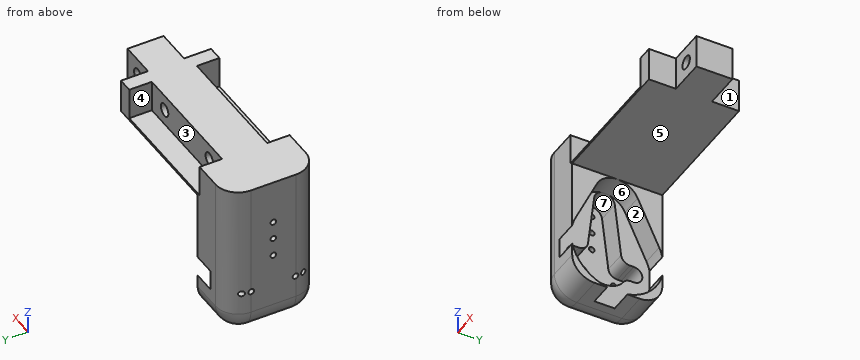
```python
from build123d import *

# Parameters (mm, degrees)
EXTRUDE_1_DEPTH      = 20
FILLET_1_R           = 5
SKETCH_2_R           = 8
CUT_EXTRUDE_1_DEPTH  = 5
SKETCH_3_R           = 6
CUT_EXTRUDE_2_DEPTH  = 1
CUT_EXTRUDE_3_DEPTH  = 5
CUT_EXTRUDE_4_DEPTH  = 5
SKETCH_6_R           = 0.625
CUT_EXTRUDE_5_DEPTH  = 4
SKETCH_7_W           = 27.5
SKETCH_7_H           = 5
CUT_EXTRUDE_6_DEPTH  = 7
SKETCH_8_R           = 1.45
CUT_EXTRUDE_7_DEPTH  = 12
CUT_EXTRUDE_8_DEPTH  = 6
CUT_EXTRUDE_START    = -20
CUT_EXTRUDE_9_DEPTH  = 6
SKETCH_13_W          = 12
SKETCH_13_H          = 27.5
CUT_EXTRUDE_10_DEPTH = 11
SKETCH_14_R          = 1.46
CUT_EXTRUDE_11_DEPTH = 11


with BuildPart() as part:
    # Эскиз1 → Бобышка-Вытянуть1 (new body)
    with BuildSketch(Plane(origin=(0, 0, 0), x_dir=(1, 0, 0), z_dir=(0, 1, 0))):
        Polygon((-13, 27.5), (-13, 0), (13, 0), (13, 27.5), (25, 27.5), (25, -7.5), (-25, -7.5), (-25, 27.5), align=None)
    extrude(amount=EXTRUDE_1_DEPTH)

    # Скругление1
    fillet_1_edges = [part.edges().sort_by_distance(p)[0] for p in [
        (19, 0, -27.5),
        (25, 10, -27.5),
        (-25, 10, -27.5),
        (-19, 20, -27.5),
        (-25, 20, -10),
        (25, 20, -10),
        (19, 20, -27.5),
        (25, 0, -10),
        (-25, 0, -10),
        (-19, 0, -27.5),
    ]]
    fillet(fillet_1_edges, radius=FILLET_1_R)

    # Эскиз2 → Вырез-Вытянуть1 (cut)
    with BuildSketch(Plane.ZY.offset(-13)):
        with Locations((-17.5, 10)):
            Circle(SKETCH_2_R)
    extrude(amount=-CUT_EXTRUDE_1_DEPTH, mode=Mode.SUBTRACT)

    # Эскиз3 → Вырез-Вытянуть2 (cut)
    with BuildSketch(Plane.ZY.offset(-18)):
        with Locations((-17.5, 10)):
            Circle(SKETCH_3_R)
    extrude(amount=-CUT_EXTRUDE_2_DEPTH, mode=Mode.SUBTRACT)

    # Эскиз4 → Вырез-Вытянуть3 (cut)
    with BuildSketch(Plane(origin=(-13, 0, 0), x_dir=(0, 0, -1), z_dir=(1, 0, 0))):
        with BuildLine():
            Line((13.195, 19.30212207), (2.9, 14.537620522))
            ThreePointArc((2.9, 14.537620522), (0, 10), (2.9, 5.462379478))
            Line((2.9, 5.462379478), (13.195, 0.69787793))
            ThreePointArc((13.195, 0.69787793), (27.75, 10), (13.195, 19.30212207))
        make_face()
    extrude(amount=-CUT_EXTRUDE_3_DEPTH, mode=Mode.SUBTRACT)

    # Эскиз5 → Вырез-Вытянуть4 (cut)
    with BuildSketch(Plane(origin=(-18, 0, 0), x_dir=(0, 0, -1), z_dir=(1, 0, 0))):
        with BuildLine():
            Line((19.4, 15.812916652), (19.4, 16.49838717))
            ThreePointArc((19.4, 16.49838717), (17.499999842, 18.39838717), (15.6, 16.498386854))
            Line((15.6, 16.498386854), (15.6, 15.665366642))
            ThreePointArc((15.6, 15.665366642), (15.094249889, 14.335999398), (13.832782732, 13.678959785))
            Line((13.832782732, 13.678959785), (1.932299859, 12.284367885))
            ThreePointArc((1.932299859, 12.284367885), (-0.1, 10), (1.932299859, 7.715632115))
            Line((1.932299859, 7.715632115), (13.832782732, 6.321040215))
            ThreePointArc((13.832782732, 6.321040215), (15.094249889, 5.664000602), (15.6, 4.334633358))
            Line((15.6, 4.334633358), (15.6, 3.501613146))
            ThreePointArc((15.6, 3.501613146), (17.5, 1.601613146), (19.4, 3.501613146))
            Line((19.4, 3.501613146), (19.4, 4.187083665))
            ThreePointArc((19.4, 4.187083665), (19.635266181, 5.128207436), (20.285714286, 5.847916677))
            ThreePointArc((20.285714286, 5.847916677), (22.5, 10), (20.285714286, 14.152083323))
            ThreePointArc((20.285714286, 14.152083323), (19.635266107, 14.871792704), (19.4, 15.812916652))
        make_face()
    extrude(amount=-CUT_EXTRUDE_4_DEPTH, mode=Mode.SUBTRACT)

    # Эскиз6 → Вырез-Вытянуть5 (cut)
    with BuildSketch(Plane(origin=(-23, 0, 0), x_dir=(0, 0, -1), z_dir=(1, 0, 0))):
        with Locations((2.278018202, 10)):
            Circle(SKETCH_6_R)
        with Locations((6.311115384, 10)):
            Circle(SKETCH_6_R)
        with Locations((10.428235425, 10)):
            Circle(SKETCH_6_R)
        with Locations((17.5, 14.907931149)):
            Circle(SKETCH_6_R)
        with Locations((17.5, 16.848859168)):
            Circle(SKETCH_6_R)
        with Locations((17.5, 5.082068851)):
            Circle(SKETCH_6_R)
        with Locations((17.5, 3.141140832)):
            Circle(SKETCH_6_R)
    extrude(amount=-CUT_EXTRUDE_5_DEPTH, mode=Mode.SUBTRACT)

    # Эскиз7 → Вырез-Вытянуть6 (cut)
    with BuildSketch(Plane.XY.offset(7.5)):
        with Locations((0, 17.5)):
            Rectangle(SKETCH_7_W, SKETCH_7_H)
        with Locations((0, 2.5)):
            Rectangle(SKETCH_7_W, SKETCH_7_H)
    extrude(amount=-CUT_EXTRUDE_6_DEPTH, mode=Mode.SUBTRACT)

    # Эскиз8 → Вырез-Вытянуть7 (cut)
    with BuildSketch(Plane(origin=(0, 15, 0), x_dir=(1, 0, 0), z_dir=(0, 1, 0))):
        with Locations(Location((-8.75, -4, 0), (0, 0, 270))):
            Circle(SKETCH_8_R)
        with Locations(Location((8.75, -4, 0), (0, 0, 270))):
            Circle(SKETCH_8_R)
    extrude(amount=-CUT_EXTRUDE_7_DEPTH, mode=Mode.SUBTRACT)

    # Эскиз11 → Вырез-Вытянуть8 (cut)
    with BuildSketch(Plane(origin=(0, 20, 0), x_dir=(1, 0, 0), z_dir=(0, 1, 0))):
        Polygon((13, 27.5), (13, 0), (17, 0), (17, -7.5), (25, -7.5), (25, 27.5), align=None)
    extrude(amount=-CUT_EXTRUDE_8_DEPTH, mode=Mode.SUBTRACT)

    # Эскиз11<2> → Вырез-Вытянуть9 (cut)
    with BuildSketch(Plane(origin=(0, 20, 0), x_dir=(1, 0, 0), z_dir=(0, 1, 0)).offset(CUT_EXTRUDE_START)):
        Polygon((13, 27.5), (13, 0), (17, 0), (17, -7.5), (25, -7.5), (25, 27.5), align=None)
    extrude(amount=CUT_EXTRUDE_9_DEPTH, mode=Mode.SUBTRACT)

    # Эскиз13 → Вырез-Вытянуть10 (cut)
    with BuildSketch(Plane(origin=(0, 14, 0), x_dir=(1, 0, 0), z_dir=(0, 1, 0))):
        with Locations((19, 13.75)):
            Rectangle(SKETCH_13_W, SKETCH_13_H)
    extrude(amount=-CUT_EXTRUDE_10_DEPTH, mode=Mode.SUBTRACT)

    # Эскиз14 → Вырез-Вытянуть11 (cut)
    with BuildSketch(Plane(origin=(0, 14, 0), x_dir=(1, 0, 0), z_dir=(0, 1, 0))):
        with Locations(Location((21, -3.75, 0), (0, 0, 270))):
            Circle(SKETCH_14_R)
    extrude(amount=-CUT_EXTRUDE_11_DEPTH, mode=Mode.SUBTRACT)


solid = part.part
```
Geometry check sheet. Reference: the model listing, model coordinates, mm. Face numbers are marked on the shaded views. A direction names the side the tool comes from. Round coordinates to 2 decimals unless told otherwise and drop trailing zeros. Order: outer loops, then holes, each group sorted by start corner. A loop starts at its lowest first (then second) coordinate and runs counter-clockwise, first axis right, second up. Notation, with made-up numbers: (57, -29.75) - (84, -29.75) arc R15 cw to (84, -9.75) - close; hole circle Ø11 at (-24, 30). An arc over 180 degrees is marked (long way). Use a Markdown table: item, result. Add a question column.
1) Section check B-B (x = 8.75). Record the cut outline in (y, z), then the cut area to 3 significant figures.
2) Thickness scan on line 1 along X through (y, z) = (8.5, 3.75); line 2 along Z through (x, y) = (-0.5, 8.25); line 3 along Y through (x, z) = (-24, -17.5). Record the ranges inside material, lowest first.
3) Mould release check, pull along X, two halves, no side actions. Record for the marked faces 1, 2 and 3: released by +X, released by -X, zero draft, split by the parting line, or undercut.
4) Section check A-A (z = -17.5). Record the cut outline in (x, y).
5) Section check C-C (z = 3.75). Count the separate pieces of the cut face and the enclosed holes in it, then the cut area to 3 significant figures.
6) Gauge pin test, flat ends, axial feed: P1, Ø2.5, axis at x = -1, y = 3, coming from the +Z side; P2, Ø5.5, axis at x = -4.5, z = 5.5, coming from the -Y side; P3, Ø1.6, axis at y = 10, z = -2.28, coming from the +X side; P4, Ø4, axis at x = 3, z = 1, coming from the -Y side. Record the tip position at first contact, or that the pin passes through.
7) Set-up check for the marked faces 4, 5, 6 and 7: record each of +Z, -Z, +X, -X, +Y, -Y from which the full face is reachable in a straight line by a thin tool's end or side.
8) Section check D-D (x = -21). Record the cut outline in (y, z).
Established:
| question | item | result |
|---|---|---|
| 1 | outline | (0, 0) - (20, 0) - (20, 0.5) - (15, 0.5) - (15, 2.55) - (5, 2.55) - (5, 0.5) - (0, 0.5) - close; (5, 5.45) - (15, 5.45) - (15, 7.5) - (5, 7.5) - close |
| 1 | area | 51.0 mm2 |
| 2 | line 1 | -25 to -10.18, -7.32 to 7.32, 10.18 to 19.54, 22.46 to 25 |
| 2 | line 2 | 0 to 7.5 |
| 2 | line 3 | 2 to 2.52, 3.77 to 4.46, 5.71 to 14.28, 15.53 to 16.22, 17.47 to 18 |
| 3 | face 1 | released by +X |
| 3 | face 2 | zero draft |
| 3 | face 3 | undercut |
| 4 | outline | (-25, 5.71) - (-23, 5.71) - (-23, 14.28) - (-25, 14.28) - close; (-24.97, 4.46) arc R5 ccw to (-24.85, 3.77) - (-23, 3.77) - (-23, 4.46) - close; (-24.97, 15.53) - (-23, 15.53) - (-23, 16.22) - (-24.85, 16.22) arc R5 ccw to start; (-24.35, 17.47) - (-23, 17.47) - (-23, 18.4) - (-18, 18.4) - (-18, 20) - (-20, 20) arc R5 ccw to start; (-24.34, 2.52) arc R5 ccw to (-20, 0) - (-18, 0) - (-18, 1.6) - (-23, 1.6) - (-23, 2.52) - close |
| 5 | separate pieces | 4 |
| 5 | enclosed holes | 0 |
| 5 | area | 538 mm2 |
| 6 | P1 | z = 0.5 |
| 6 | P2 | y = 5 |
| 6 | P3 | x = -23 |
| 6 | P4 | y = 0 |
| 7 | face 4 | +Z, +Y |
| 7 | face 5 | -Z, +X, +Y, -Y |
| 7 | face 6 | +X |
| 7 | face 7 | none |
| 8 | outline | (0.1, -22.5) arc R4.9 ccw to (5, -27.4) - (15, -27.4) arc R4.9 ccw to (19.9, -22.5) - (19.9, 7.5) - (0.1, 7.5) - close; hole (3.5, -19.4) - (4.19, -19.4) arc R2 cw to (5.85, -20.29) arc R5 ccw to (14.15, -20.29) arc R2 cw to (15.81, -19.4) - (16.5, -19.4) arc R1.9 ccw to (16.5, -15.6) - (15.67, -15.6) arc R2 cw to (13.68, -13.83) - (12.28, -1.93) arc R2.3 ccw to (7.72, -1.93) - (6.32, -13.83) arc R2 cw to (4.33, -15.6) - (3.5, -15.6) arc R1.9 ccw to start |
